Design review of the part built by this model. Coordinates are the model's own, in mm. A direction names the side the tool comes from. Coordinates: 2 decimals unless noted, no trailing zeros. Loops run counter-clockwise (first coordinate to the right, second up) from the corner with the lowest first, then second, coordinate; pieces in that order, holes last. Notation, with made-up numbers: M 76.5,4 L 122.5,4 A9 ccw 122.5,15 Z; hole C 87.25,57.5 d7. An arc over 180 degrees is marked long. Answer as a JSON object with one key per item and string values. Group by question number.
1. To check wall thickness, follow probe 1 along Y at (x, z) = (25, -62.95); probe 2 along Y at (x, z) = (88, 63.3); probe 3 along Y at (x, z) = (85, 63). State the ranges of each line that lie inside material, in increasing order.
2. Consider section B-B (y = 39.5). State the section outline as (x, z) points, then the cut area to 3 significant figures.
3. Insertion check: pin 1 (5 mm diameter, centred on y = -23.5, z = 30.5, fed in from +X). The pin has a flat end and moves straight along its axis. Give the tip position at first contact, or say it passes through.
4. Consider section A-A (x = 63). State the section outline as (y, z) points.
5. Draft analysis for pull direction Z (two halves, no side actions). For faces 1 (the flat face through (47, 3, 64.5)), 2 (the flat face through (49, 3, 62.5)), 3 (the flat face through (47, -3, -64.5)), state which applies: +Z half, -Z half, draft (parallel to the pull), parting line (faces both ways), or undercut.
6. Machinability: for faces 4 (the flat face through (-2, -3, 1)), 5 (the flat face through (0, -3, 1)), which of the approach directions +Z, -Z, +X, -X, +Y, -Y give a long, thin tool a straight path to every point of the face, cutting with its end or side? Answer none if there is none.
7. Consider section C-C (z = -1.5). State the section outline as (x, y) points.
from build123d import *

# Parameters (mm, degrees)
SKETCH1_W                      = 370
SKETCH1_H                      = 129
SKETCH1_R                      = 1.6
BASE_FLANGE2_DEPTH             = 2
EDGE_FLANGE2_STRIP_W           = 9.9304
EDGE_FLANGE2_STRIP_H           = 2
EDGE_FLANGE2_STRIP_CUT_DEPTH   = 370
EDGE_FLANGE2_STRIP_2_W         = 9.9304
EDGE_FLANGE2_STRIP_2_H         = 2
EDGE_FLANGE2_STRIP_CUT_2_DEPTH = 370
EDGE_FLANGE2_DEPTH             = 370
EDGE_FLANGE2_BEND_DEPTH        = 370
SKETCH23_R                     = 1.6
CUT_EXTRUDE2_DEPTH             = 245.726377818


# Sheet-metal steps are written as plain solids
with BuildPart() as part:
    # Sketch1 → Base-Flange2 (new body)
    with BuildSketch(Plane.YZ):
        Rectangle(SKETCH1_W, SKETCH1_H)
        with Locations(Location((-170, 57.5, 0), (0, 0, 270))):
            Circle(SKETCH1_R, mode=Mode.SUBTRACT)
        with Locations(Location((137.3, 57.5, 0), (0, 0, 270))):
            Circle(SKETCH1_R, mode=Mode.SUBTRACT)
        with Locations(Location((-170, -57.5, 0), (0, 0, 270))):
            Circle(SKETCH1_R, mode=Mode.SUBTRACT)
        with Locations(Location((137.3, -57.5, 0), (0, 0, 270))):
            Circle(SKETCH1_R, mode=Mode.SUBTRACT)
        with Locations(Location((34.3, 57.5, 0), (0, 0, 270))):
            Circle(SKETCH1_R, mode=Mode.SUBTRACT)
        with Locations(Location((-12.7, -57.5, 0), (0, 0, 270))):
            Circle(SKETCH1_R, mode=Mode.SUBTRACT)
    extrude(amount=-BASE_FLANGE2_DEPTH)

    # Edge-Flange2 strip (across the edge) → Edge-Flange2 strip cut (cut)
    with BuildSketch(Plane(origin=(0, -185, -64.5), x_dir=(0, 0, 1), z_dir=(0, 1, 0))):
        with Locations((-2, -1)):
            Rectangle(EDGE_FLANGE2_STRIP_W, EDGE_FLANGE2_STRIP_H)
    extrude(amount=EDGE_FLANGE2_STRIP_CUT_DEPTH, mode=Mode.SUBTRACT)

    # Edge-Flange2 strip 2 (across the edge) → Edge-Flange2 strip cut 2 (cut)
    with BuildSketch(Plane(origin=(0, 185, 64.5), x_dir=(0, 0, -1), z_dir=(0, -1, 0))):
        with Locations((-2, -1)):
            Rectangle(EDGE_FLANGE2_STRIP_2_W, EDGE_FLANGE2_STRIP_2_H)
    extrude(amount=EDGE_FLANGE2_STRIP_CUT_2_DEPTH, mode=Mode.SUBTRACT)

    # Edge-Flange2 section (across the edge) → Edge-Flange2 (add)
    with BuildSketch(Plane(origin=(0, -185, -64.5), x_dir=(0, 0, 1), z_dir=(0, 1, 0))):
        with BuildLine():
            Line((0, 0.9652), (0, 95))
            Line((0, 95), (2, 95))
            Line((2, 95), (2, 0.9652))
            ThreePointArc((2, 0.9652), (2.282700535, 0.282700535), (2.9652, 0))
            Line((2.9652, 0), (2.9652, -2))
            ThreePointArc((2.9652, -2), (0.868486972, -1.131513028), (0, 0.9652))
        make_face()
    extrude(amount=EDGE_FLANGE2_DEPTH)

    # Edge-Flange2 section 2 (across the edge) → Edge-Flange2 bend (add)
    with BuildSketch(Plane(origin=(0, 185, 64.5), x_dir=(0, 0, -1), z_dir=(0, -1, 0))):
        with BuildLine():
            Line((0, 0.9652), (0, 95))
            Line((0, 95), (2, 95))
            Line((2, 95), (2, 0.9652))
            ThreePointArc((2, 0.9652), (2.282700535, 0.282700535), (2.9652, 0))
            Line((2.9652, 0), (2.9652, -2))
            ThreePointArc((2.9652, -2), (0.868486972, -1.131513028), (0, 0.9652))
        make_face()
    extrude(amount=EDGE_FLANGE2_BEND_DEPTH)

    # Sketch23 → Cut-Extrude2 (cut, through all)
    with BuildSketch(Plane(origin=(0, 0, -64.5), x_dir=(1, 0, 0), z_dir=(0, 0, -1))):
        with Locations(Location((88, 150, 0), (0, 0, 180))):
            Circle(SKETCH23_R)
        with Locations(Location((88, 0, 0), (0, 0, 180))):
            Circle(SKETCH23_R)
        with Locations(Location((88, -150, 0), (0, 0, 180))):
            Circle(SKETCH23_R)
        with Locations(Location((8, 180, 0), (0, 0, 180))):
            Circle(SKETCH23_R)
        with Locations(Location((85, 180, 0), (0, 0, 180))):
            Circle(SKETCH23_R)
        with Locations(Location((8, -180, 0), (0, 0, 180))):
            Circle(SKETCH23_R)
        with Locations(Location((85, -180, 0), (0, 0, 180))):
            Circle(SKETCH23_R)
        with Locations(Location((25, -15, 0), (0, 0, 180))):
            Circle(SKETCH23_R)
        with Locations(Location((25, 51.5, 0), (0, 0, 180))):
            Circle(SKETCH23_R)
    extrude(amount=-CUT_EXTRUDE2_DEPTH, mode=Mode.SUBTRACT)


solid = part.part
Findings below:
{
 "1": {"probe 1": "y = -185 to -53.1, -49.9 to 13.4, 16.6 to 185", "probe 2": "y = -185 to -151.6, -148.4 to -1.6, 1.6 to 148.4, 151.6 to 185", "probe 3": "y = -185 to -181.6, -178.4 to 178.4, 181.6 to 185"},
 "2": {"outline": "M -2,-61.53 A2.97 ccw 0.97,-64.5 L 95,-64.5 L 95,-62.5 L 0.97,-62.5 A0.97 cw 0,-61.53 L 0,61.53 A0.97 cw 0.97,62.5 L 95,62.5 L 95,64.5 L 0.97,64.5 A2.97 ccw -2,61.53 Z", "area": "635 mm^2"},
 "3": {"pin 1": "stops at x = 0"},
 "4": {"outline": "M -185,-64.5 L 185,-64.5 L 185,-62.5 L -185,-62.5 Z; M -185,62.5 L 185,62.5 L 185,64.5 L -185,64.5 Z"},
 "5": {"face 1": "+Z half", "face 2": "undercut", "face 3": "-Z half"},
 "6": {"face 4": "+Z, -Z, -X, +Y, -Y", "face 5": "+X, +Y, -Y"},
 "7": {"outline": "M -2,-185 L 0,-185 L 0,185 L -2,185 Z"}
}
